Autodesk Inventor part; units mm, degrees
ref_plane "YZ Plane" through (0, 0, 0) normal (1, 0, 0) x (0, 1, 0)
ref_plane "XZ Plane" through (0, 0, 0) normal (0, 1, 0) x (-1, 0, 0)
ref_plane "XY Plane" through (0, 0, 0) normal (0, 0, 1) x (1, 0, 0)
sketch "Sketch1" plane through (0, 0, 0) normal (0, 0, 1) x (1, 0, 0)
  line L0 (0, 0) -> (542, 0)
  line L1 (542, 0) -> (542, 350)
  line L2 (0, 350) -> (0, 0)
  line L3 (271, 0) -> (271, 353)
  arc A0 (193.5581, 350) -> (348.4419, 350) centre (271, 353) ccw
  line L4 (542, 350) -> (348.4419, 350)
  line L5 (193.5581, 350) -> (0, 350)
  dimension "d0" = 542
  dimension "d1" = 350
  dimension "d24" = 155
  dimension "d25" = 353
extrude "Extrusion1" add sketch "Sketch1" along normal blind 3
sketch "Sketch2" plane through (0, 0, 0) normal (0, 0, -1) x (-1, 0, 0)
  line L0 (0, 350) -> (0, 0)
  line L1 (-542, 0) -> (-542, 350)
  line L2 (-542, 350) -> (0, 350)
  point P0 (-23, 330)
  point P1 (-23, 20)
  point P2 (-519, 330)
  point P3 (-519, 20)
  dimension "d4" = 23
  dimension "d13" = 20
  dimension "d14" = 350
  dimension "d15" = 542
  dimension "d18" = 310
  dimension "d21" = 496
hole "Hole1" at (23, 330, 0) at (519, 330, 0) at (519, 20, 0) at (23, 20, 0) direction (0, 0, 1) diameter 6.5 end through all
properties part number "plate_top_02" material "Polystyrene"
Geometry: final body of the model. Coordinates: model frame, mm. Coordinates: 2 decimals unless noted, no trailing zeros. Order: outer loops, then holes, each group sorted by start corner. A loop starts at its lowest first (then second) coordinate and runs counter-clockwise, first axis right, second up. Notation, with made-up numbers: M 71.5,-29.75 L 82.5,-29.75 A24 ccw 82.5,-1.75 Z; hole C 10.25,-28 d11. An arc over 180 degrees is marked long. Answer as CSV lines item,"result".
Q1. Line query: probe 1 along Y at (x, z) = (23, 1.4); probe 2 along X at (y, z) = (20, 1.8); probe 3 along X at (y, z) = (330, 1.9). Output: solid intervals per line, ascending. Write a range as [from, to].
Answers:
probe 1,"y = [0, 16.75], [23.25, 326.75], [333.25, 350]"
probe 2,"x = [0, 19.75], [26.25, 515.75], [522.25, 542]"
probe 3,"x = [0, 19.75], [26.25, 196.99], [345.01, 515.75], [522.25, 542]"
Q2. Section B-B on z = 0.55. Return the cut outline in (x, y).
Answers:
outline,"M 0,0 L 542,0 L 542,350 L 348.44,350 A77.5 cw 193.56,350 L 0,350 Z; hole C 23,20 d6.5; hole C 23,330 d6.5; hole C 519,20 d6.5; hole C 519,330 d6.5"
Q3. First-contact query: P1, Ø1, axis at x = 83.5, z = 2.5, coming from the -Y side. Flat tip, straight axial feed; report the tip coordinate or a pass-through.
Answers:
P1,"stops at y = 0"
Q4. Section A-A on y = 289. Return the cut outline in (x, z).
Answers:
outline,"M 0,0 L 227.29,0 L 227.29,3 L 0,3 Z; M 314.71,0 L 542,0 L 542,3 L 314.71,3 Z"
Q5. Section C-C on x = 271. Return the cut outline in (y, z), and give its area (4 significant figures).
Answers:
outline,"M 0,0 L 275.5,0 L 275.5,3 L 0,3 Z"
area,"826.5 mm^2"
Q6. Draft query along X for faces 1 (the cylindrical face through (272.662, 275.518, 1.479)), 2 (the flat face through (267, 177, 3)). Return one class per face: pulls with the +X half, pulls with the -X half, needs draft (parallel to the pull), parting line crosses it, or undercut.
Answers:
face 1,"undercut"
face 2,"needs draft"
